from build123d import *

# Parameters (mm, degrees)
ESQUISSE1_R                                   = 12
BOSS_EXTRU_1_DEPTH                            = 1
ESQUISSE2_R                                   = 24
BOSS_EXTRU_2_DEPTH                            = 6
TROU_POUR_TARAUDAGE_POUR_TROU_TARAUD_M4_D     = 3.3
TROU_POUR_TARAUDAGE_POUR_TROU_TARAUD_M4_DEPTH = 6
TROU_POUR_TARAUDAGE_POUR_TROU_TARAUD_M4_TIP   = 0.991420021
ESQUISSE12_R                                  = 5
BOSS_EXTRU_3_DEPTH                            = 56
TROU_POUR_TARAUDAGE_POUR_TROU_TARAUD_M5_D     = 4.2
TROU_POUR_TARAUDAGE_POUR_TROU_TARAUD_M5_DEPTH = 20
TROU_POUR_TARAUDAGE_POUR_TROU_TARAUD_M5_TIP   = 1.2618073
ENL_V_START                                   = 3.2
ENL_V_MAT_EXTRU_3_DEPTH                       = 21.8
ESQUISSE19_R                                  = 10
BOSS_EXTRU_4_DEPTH                            = 7


with BuildPart() as part:
    # Esquisse1 → Boss.-Extru.1 (new body)
    with BuildSketch(Plane.XY):
        Circle(ESQUISSE1_R)
    extrude(amount=BOSS_EXTRU_1_DEPTH)

    # Esquisse2 → Boss.-Extru.2 (add)
    with BuildSketch(Plane(origin=(0, 0, 0), x_dir=(-1, 0, 0), z_dir=(0, 0, -1))):
        Circle(ESQUISSE2_R)
    extrude(amount=BOSS_EXTRU_2_DEPTH)

    # Trou pour taraudage pour trou taraudé M42
    with Locations(Plane(origin=(0, 0, -6), x_dir=(-1, 0, 0), z_dir=(0, 0, -1))):
        with Locations((-17, 9), (17, -9), (17, 9), (-17, -9)):
            Hole(TROU_POUR_TARAUDAGE_POUR_TROU_TARAUD_M4_D / 2, depth=TROU_POUR_TARAUDAGE_POUR_TROU_TARAUD_M4_DEPTH)
            with Locations((0, 0, -(TROU_POUR_TARAUDAGE_POUR_TROU_TARAUD_M4_DEPTH + TROU_POUR_TARAUDAGE_POUR_TROU_TARAUD_M4_TIP / 2))):  # 118° drill point
                Cone(0, TROU_POUR_TARAUDAGE_POUR_TROU_TARAUD_M4_D / 2, TROU_POUR_TARAUDAGE_POUR_TROU_TARAUD_M4_TIP, mode=Mode.SUBTRACT)

    # Esquisse12 → Boss.-Extru.3 (add)
    with BuildSketch(Plane.XY.offset(1)):
        Circle(ESQUISSE12_R)
    extrude(amount=BOSS_EXTRU_3_DEPTH)

    # Trou pour taraudage pour trou taraudé M51
    with Locations(Plane.XY.offset(57)):
        with Locations((0, 0)):
            Hole(TROU_POUR_TARAUDAGE_POUR_TROU_TARAUD_M5_D / 2, depth=TROU_POUR_TARAUDAGE_POUR_TROU_TARAUD_M5_DEPTH)
            with Locations((0, 0, -(TROU_POUR_TARAUDAGE_POUR_TROU_TARAUD_M5_DEPTH + TROU_POUR_TARAUDAGE_POUR_TROU_TARAUD_M5_TIP / 2))):  # 118° drill point
                Cone(0, TROU_POUR_TARAUDAGE_POUR_TROU_TARAUD_M5_D / 2, TROU_POUR_TARAUDAGE_POUR_TROU_TARAUD_M5_TIP, mode=Mode.SUBTRACT)

    # Esquisse16 → Enlèv. mat.-Extru.3 (cut, through all)
    with BuildSketch(Plane(origin=(0, 0, 0), x_dir=(1, 0, 0), z_dir=(0, 1, 0)).offset(ENL_V_START)):
        with BuildLine():
            Line((-1.5, -57), (-1.5, -32.669951792))
            ThreePointArc((-1.5, -32.669951792), (0, -31.169951792), (1.5, -32.669951792))
            Line((1.5, -32.669951792), (1.5, -57))
            ThreePointArc((1.5, -57), (0, -58.5), (-1.5, -57))
        make_face()
    extrude(amount=ENL_V_MAT_EXTRU_3_DEPTH, mode=Mode.SUBTRACT)

    # Esquisse19 → Boss.-Extru.4 (add)
    with BuildSketch(Plane.XY.offset(1)):
        Circle(ESQUISSE19_R)
    extrude(amount=BOSS_EXTRU_4_DEPTH)


solid = part.part
Source: CAD feature listing. Evaluate the final solid. Frame: model axes, mm. A direction names the side the tool comes from. Give positions to 0.01 mm unless a question says otherwise; leave off trailing zeros. Write each loop counter-clockwise with the first axis right and the second up, starting at its lowest first coordinate (ties: lowest second). Pieces come first, ordered by that corner, then holes. Notation, with made-up numbers: (-19.75, -16) -> (16.25, -16) arc R17 cw to (16.25, -9) -> close; hole circle Ø6 at (17, 80). An arc over 180 degrees is marked (long way). Return JSON: item names as keys, results as strings. Group by question number.
1. Material intervals for line 1 (X direction, y = 0, z = 47.5); line 2 (Y direction, x = 0, z = 48); line 3 (X direction, y = -9, z = -4), sorted ascending. Write a range as from..to.
2. Section C-C, the plane y = -9. Output: boundary loops of the cut face in (x, z), then the cut area to 3 significant figures.
3. Section A-A, the plane z = 42. Output: boundary loops of the cut face in (x, y), then the cut area to 3 significant figures.
4. Section D-D, the plane x = 7. Output: boundary loops of the cut face in (y, z), then the cut area to 3 significant figures.
5. Pin query (flat end, axial travel): pin 1 Ø0.8 at (y, z) = (4.5, 40.5) entering from +X; pin 2 Ø2 at (x, y) = (-17, -9) entering from -Z; pin 3 Ø10 at (y, z) = (11, 9.5) entering from +X; pin 4 Ø3 at (y, z) = (-3.5, 15) entering from +X. Return the tip coordinate at first contact, or that it passes through.
6. Section B-B, the plane x = 17. Output: boundary loops of the cut face in (y, z).
7. Mould query, pull axis Y, two halves, no side actions, for faces 4 (the face through (0.35, 0.11, 35.96)), 5 (the face through (1, -2.2, 57)), 6 (the face through (-1.08, -4.88, 32.16)). Classes: +Y half, -Y half, draft (parallel to the pull), parting line (faces both ways), or undercut.
8. Access query for faces 1 (the face through (6, 11, 0)), 2 (the face through (0, 3.2, 44)), 3 (the face through (-15.476, 8.368, -2.958)). Directions: +Z, -Z, +X, -X, +Y, -Y. A direction counts if a zero-diameter tool reaches every point of the face in a straight line with its end or side. Return the directions, or none.
Determined:
{
 "1": {"line 1": "x = -5..-2.1, 2.1..5", "line 2": "y = -5..-2.1, 2.1..3.2", "line 3": "x = -22.25..-18.65, -15.35..15.35, 18.65..22.25"},
 "2": {"outline": "(-22.25, -6) -> (-18.65, -6) -> (-18.65, 0) -> (-22.25, 0) -> close; (-15.35, -6) -> (15.35, -6) -> (15.35, 0) -> (7.94, 0) -> (7.94, 1) -> (4.36, 1) -> (4.36, 8) -> (-4.36, 8) -> (-4.36, 1) -> (-7.94, 1) -> (-7.94, 0) -> (-15.35, 0) -> close; (18.65, -6) -> (22.25, -6) -> (22.25, 0) -> (18.65, 0) -> close", "area": "304 mm2"},
 "3": {"outline": "(-1.5, 3.2) -> (-1.5, 4.77) arc R5 ccw (long way) to (1.5, 4.77) -> (1.5, 3.2) -> close; hole circle Ø4.2 at (0, 0)", "area": "59.5 mm2"},
 "4": {"outline": "(-22.96, -6) -> (22.96, -6) -> (22.96, 0) -> (9.75, 0) -> (9.75, 1) -> (7.14, 1) -> (7.14, 8) -> (-7.14, 8) -> (-7.14, 1) -> (-9.75, 1) -> (-9.75, 0) -> (-22.96, 0) -> close", "area": "395 mm2"},
 "5": {"pin 1": "stops at x = 2.86", "pin 2": "passes through", "pin 3": "stops at x = 7.82", "pin 4": "stops at x = 4.58"},
 "6": {"outline": "(-16.94, -6) -> (-10.65, -6) -> (-10.65, 0) -> (-16.94, 0) -> close; (-7.35, -6) -> (7.35, -6) -> (7.35, 0) -> (-7.35, 0) -> close; (10.65, -6) -> (16.94, -6) -> (16.94, 0) -> (10.65, 0) -> close"},
 "7": {"face 4": "undercut", "face 5": "draft", "face 6": "parting line"},
 "8": {"face 1": "+Z", "face 2": "+Z, +Y", "face 3": "+Z, -Z"}
}
